Geometry: see drawing. Coordinates: mm, zero at the bounding-box minimum. Round coordinates to 2 decimals unless told otherwise and drop trailing zeros. Loops run counter-clockwise (first coordinate to the right, second up) from the corner with the lowest first, then second, coordinate; pieces in that order, holes last.
(1) Cut plane B-B, the plane y = 86. Output: boundary loops of the cut face in (x, z) (3 decimals), and give its area (3 significant figures).
(2) First-contact query: pin 1 Ø1 at (x, z) = (329.5, 1.5) entering from +Y (3 decimals); pin 2 Ø1.6 at (x, z) = (316, 1.5) entering from -Y (3 decimals); pin 3 Ø1.5 at (y, z) = (19, 2.5) entering from +X (3 decimals). Flat tips, straight axial feed; report the tip coordinate or a pass-through.
(3) Cut plane C-C, the plane x = 177. Output: boundary loops of the cut face in (y, z) (3 decimals), and give its area (3 significant figures).
(4) Cut plane A-A, the plane z = 1.6. Give the number of separate pieces and of enclosed holes in the cut face, and give its area (3 significant figures).
(5) Line query: line 1 (X direction, y = 25.5, z = 0.4) (3 decimals); line 2 (X direction, y = 78, z = 1.35) (3 decimals); line 3 (Y direction, x = 311.5, z = 1.25) (3 decimals). Output: solid intervals per line, ascending.
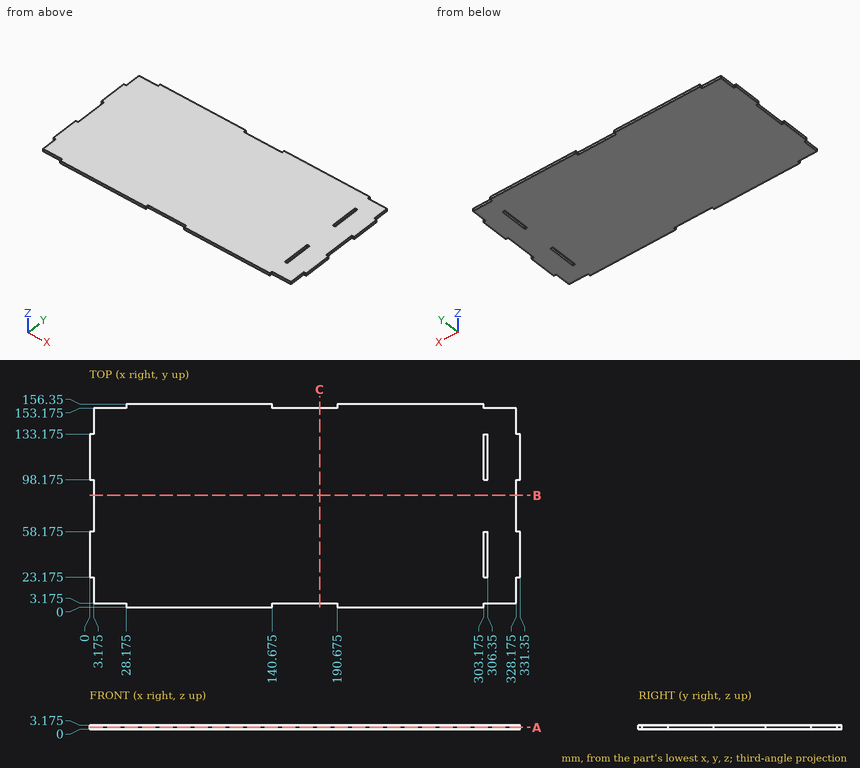
Reported:
1. outline: (3.175, 0) - (328.175, 0) - (328.175, 3.175) - (3.175, 3.175) - close
1. area: 1,030 mm2
2. pin 1: stops at y = 133.175
2. pin 2: stops at y = 3.175
2. pin 3: stops at x = 328.175
3. outline: (3.175, 0) - (153.175, 0) - (153.175, 3.175) - (3.175, 3.175) - close
3. area: 476 mm2
4. separate pieces: 1
4. enclosed holes: 2
4. area: 50,400 mm2
5. line 1: x = 0 to 303.175, 306.35 to 331.35
5. line 2: x = 3.175 to 328.175
5. line 3: y = 3.175 to 153.175
